The model under review builds one solid part; all positions refer to its coordinate system, in mm. A direction names the side the tool comes from. Round coordinates to 2 decimals unless told otherwise and drop trailing zeros. Loops run counter-clockwise (first coordinate to the right, second up) from the corner with the lowest first, then second, coordinate; pieces in that order, holes last. Notation, with made-up numbers: (10.25, 38) -> (40.25, 38) arc R24 cw to (40.25, 66) -> close; hole circle Ø5 at (-39, 36). An arc over 180 degrees is marked (long way). Return JSON: item names as keys, results as strings. Group by question number.
```python
from build123d import *

# Parameters (mm, degrees)
SKETCH1_W           = 20
SKETCH1_H           = 50
SKETCH1_R           = 1.75
SKETCH1_R_2         = 2.25
SKETCH1_R_3         = 2.5
SKETCH1_R_4         = 7
SKETCH1_W_2         = 8
SKETCH1_H_2         = 4.5
SKETCH1_W_3         = 5
SKETCH1_H_3         = 2.85
BOSS_EXTRUDE1_DEPTH = 3


with BuildPart() as part:
    # Sketch1 → Boss-Extrude1 (new body)
    with BuildSketch(Plane.XY):
        with Locations((10, 25)):
            Rectangle(SKETCH1_W, SKETCH1_H)
        with Locations((16.25, 23.75)):
            Circle(SKETCH1_R, mode=Mode.SUBTRACT)
        with Locations((15.75, 45.75)):
            Circle(SKETCH1_R_2, mode=Mode.SUBTRACT)
        with Locations((10, 10)):
            Circle(SKETCH1_R_3, mode=Mode.SUBTRACT)
        with Locations((10, 35)):
            Circle(SKETCH1_R_4, mode=Mode.SUBTRACT)
        with Locations((6, 45.75)):
            Rectangle(SKETCH1_W_2, SKETCH1_H_2, mode=Mode.SUBTRACT)
        with Locations((10, 2.425)):
            Rectangle(SKETCH1_W_3, SKETCH1_H_3, mode=Mode.SUBTRACT)
        with Locations((10, 17.575)):
            Rectangle(SKETCH1_W_3, SKETCH1_H_3, mode=Mode.SUBTRACT)
    extrude(amount=BOSS_EXTRUDE1_DEPTH)


solid = part.part
```
1. We need section B-B, the plane z = 1.7. Write out the cut boundary in (x, y).
2. Draft analysis for pull direction X (two halves, no side actions). For faces 1 (the face through (7.5, 18, 1)), 2 (the face through (10, 25, 3)), state which applies: pulls with the +X half, pulls with the -X half, needs draft (parallel to the pull), parting line crosses it, or undercut.
3. We need section A-A, the plane y = 10. Write out the cut boundary in (x, z).
4. Wall thickness on line 1 (Y direction, x = 2.5, z = 2.1); line 2 (Y direction, x = 9.5, z = 1.35); line 3 (Y direction, x = 15.75, z = 0.9): over which ranges is each line inside the solid? List them lowest first.
5. We need section D-D, the plane y = 45.75. Write out the cut boundary in (x, z).
6. For P1, Ø2, axis at x = 16.25, y = 23.75, coming from the +Z side, flat-tipped, find the tip position at first contact; note if it passes through.
7. We need section C-C, the plane x = 7. Write out the cut boundary in (y, z).
8. Tool access review of faces 3 (the face through (10, 50, 1)), 4 (the face through (12.5, 18, 1)): name each direction out of +Z, -Z, +X, -X, +Y, -Y from which nothing blocks a thin tool from reaching the whole face with its end or side.
Check sheet entries:
{
 "1": {"outline": "(0, 0) -> (20, 0) -> (20, 50) -> (0, 50) -> close; hole (2, 43.5) -> (10, 43.5) -> (10, 48) -> (2, 48) -> close; hole circle Ø14 at (10, 35); hole (7.5, 1) -> (12.5, 1) -> (12.5, 3.85) -> (7.5, 3.85) -> close; hole circle Ø5 at (10, 10); hole (7.5, 16.15) -> (12.5, 16.15) -> (12.5, 19) -> (7.5, 19) -> close; hole circle Ø4.5 at (15.75, 45.75); hole circle Ø3.5 at (16.25, 23.75)"},
 "2": {"face 1": "undercut", "face 2": "needs draft"},
 "3": {"outline": "(0, 0) -> (7.5, 0) -> (7.5, 3) -> (0, 3) -> close; (12.5, 0) -> (20, 0) -> (20, 3) -> (12.5, 3) -> close"},
 "4": {"line 1": "y = 0 to 43.5, 48 to 50", "line 2": "y = 0 to 1, 3.85 to 7.55, 12.45 to 16.15, 19 to 28.02, 41.98 to 43.5, 48 to 50", "line 3": "y = 0 to 22.07, 25.43 to 31.01, 38.99 to 43.5, 48 to 50"},
 "5": {"outline": "(0, 0) -> (2, 0) -> (2, 3) -> (0, 3) -> close; (10, 0) -> (13.5, 0) -> (13.5, 3) -> (10, 3) -> close; (18, 0) -> (20, 0) -> (20, 3) -> (18, 3) -> close"},
 "6": {"P1": "passes through"},
 "7": {"outline": "(0, 0) -> (28.68, 0) -> (28.68, 3) -> (0, 3) -> close; (41.32, 0) -> (43.5, 0) -> (43.5, 3) -> (41.32, 3) -> close; (48, 0) -> (50, 0) -> (50, 3) -> (48, 3) -> close"},
 "8": {"face 3": "+Z, -Z, +X, -X, +Y", "face 4": "+Z, -Z"}
}
